Check sheet for the drawn part. Datum: minimum x, y, z corner. Units: mm. A direction names the side the tool comes from. Give positions to 0.01 mm unless a question says otherwise; leave off trailing zeros. Order: outer loops, then holes, each group sorted by start corner. A loop starts at its lowest first (then second) coordinate and runs counter-clockwise, first axis right, second up.
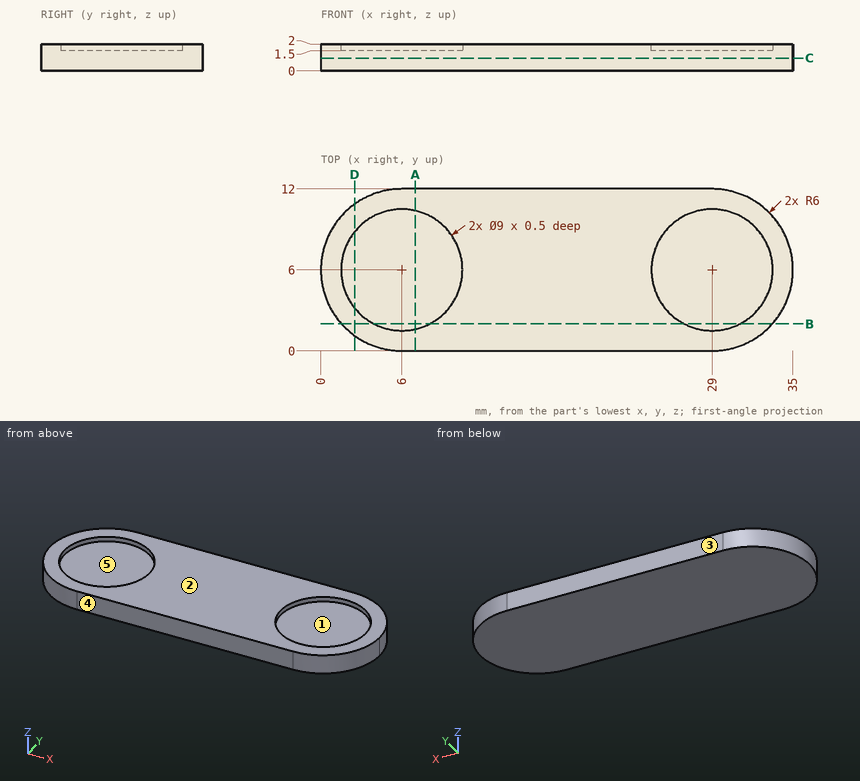
(1) Section check B-B, the plane y = 2. Enter the section's corners in (x, z), then the cut area to 3 significant figures.
Solved:
outline: (1.53, 0) - (33.47, 0) - (33.47, 2) - (31.06, 2) - (31.06, 1.5) - (26.94, 1.5) - (26.94, 2) - (8.06, 2) - (8.06, 1.5) - (3.94, 1.5) - (3.94, 2) - (1.53, 2) - close
area: 59.8 mm2
(2) Go/stop test with a flat-tipped pin: pin 1 (4.5 mm diameter, centred on x = 6, y = 4, fed in from +Z). Record where the tip stops, or that it passes through.
Solved:
pin 1: stops at z = 1.5
(3) Section check A-A, the plane x = 7. Enter the section's corners in (y, z).
Solved:
outline: (0, 0) - (12, 0) - (12, 2) - (10.39, 2) - (10.39, 1.5) - (1.61, 1.5) - (1.61, 2) - (0, 2) - close
(4) Release check for a two-part mould opening along Y. For the marked faces 3, 4 and 5 record: pulls with the +Y half, pulls with the -Y half, needs draft (parallel to the pull), parting line crosses it, or undercut.
Solved:
face 3: pulls with the +Y half
face 4: pulls with the -Y half
face 5: undercut
(5) Scan lines: line 1 (Y direction, x = 6, z = 1.7); line 2 (Z direction, x = 31, y = 3); line 3 (Y direction, x = 7, z = 1.65). Record each from-to range of solid material in increasing order.
Solved:
line 1: y = 0 to 1.5, 10.5 to 12
line 2: z = 0 to 1.5
line 3: y = 0 to 1.61, 10.39 to 12
(6) Set-up check for the marked faces 1 and 2: record each of +Z, -Z, +X, -X, +Y, -Y from which the full face is reachable in a straight line by a thin tool's end or side.
Solved:
face 1: +Z
face 2: +Z, +X, -X, +Y, -Y
(7) Section check C-C, the plane z = 0.95. Enter the section's corners in (x, y), then the cut area to 3 significant figures.
Solved:
outline: (6, 0) - (29, 0) arc R6 ccw to (35, 6) arc R6 ccw to (29, 12) - (6, 12) arc R6 ccw to start
area: 389 mm2
(8) Section check D-D, the plane x = 2.5. Enter the section's corners in (y, z), then the cut area to 3 significant figures.
Solved:
outline: (1.13, 0) - (10.87, 0) - (10.87, 2) - (8.83, 2) - (8.83, 1.5) - (3.17, 1.5) - (3.17, 2) - (1.13, 2) - close
area: 16.7 mm2
